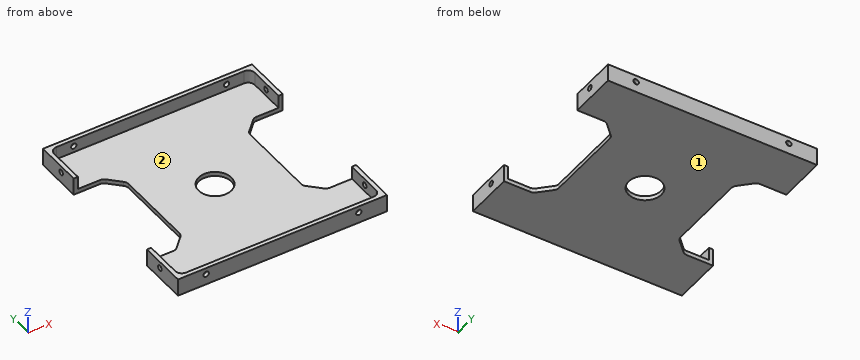
```python
from build123d import *

# Parameters (mm, degrees)
SKETCH1_W                      = 95.8
SKETCH1_H                      = 95.8
BOSS_EXTRUDE1_DEPTH            = 8
SKETCH2_W                      = 92
SKETCH2_H                      = 92
COMPONENT_PLATFORM_DEPTH       = 6
CABLE_SLOTS_DEPTH              = 6
SKETCH4_R                      = 7.5
CENTER_MASS_CUT_DEPTH          = 6
INNER_CORNER_FILLETS_R         = 3
M3X0_5_TAPPED_HOLE1_AT_2_COUNT = 2
M3X0_5_TAPPED_HOLE1_AT_2_PITCH = 70
M3X0_5_TAPPED_HOLE2_AT_2_COUNT = 2
M3X0_5_TAPPED_HOLE2_AT_2_PITCH = 70


with BuildPart() as part:
    # Sketch1 → Boss-Extrude1 (new body)
    with BuildSketch(Plane.XY):
        Rectangle(SKETCH1_W, SKETCH1_H)
    extrude(amount=BOSS_EXTRUDE1_DEPTH)

    # Sketch2 → Component Platform (cut)
    with BuildSketch(Plane.XY.offset(8)):
        Rectangle(SKETCH2_W, SKETCH2_H)
    extrude(amount=-COMPONENT_PLATFORM_DEPTH, mode=Mode.SUBTRACT)

    # Sketch3 → Cable Slots (cut, symmetric)
    with BuildSketch(Plane.XY.offset(2)):
        with BuildLine():
            Line((-33.778679656, -25.021320344), (-28.778679656, -20.021320344))
            ThreePointArc((-28.778679656, -20.021320344), (-28.128361402, -19.048050297), (-27.9, -17.9))
            Line((-27.9, -17.9), (-27.9, 18.1))
            ThreePointArc((-27.9, 18.1), (-28.128361402, 19.248050297), (-28.778679656, 20.221320344))
            Line((-28.778679656, 20.221320344), (-33.778679656, 25.221320344))
            ThreePointArc((-33.778679656, 25.221320344), (-34.751949703, 25.871638598), (-35.9, 26.1))
            Line((-35.9, 26.1), (-47.9, 26.1))
            Line((-47.9, 26.1), (-47.9, -25.9))
            Line((-47.9, -25.9), (-35.9, -25.9))
            ThreePointArc((-35.9, -25.9), (-34.751949703, -25.671638598), (-33.778679656, -25.021320344))
        make_face()
        with BuildLine():
            Line((47.9, -25.9), (47.9, 26.1))
            Line((47.9, 26.1), (35.9, 26.1))
            ThreePointArc((35.9, 26.1), (34.751949703, 25.871638598), (33.778679656, 25.221320344))
            Line((33.778679656, 25.221320344), (28.778679656, 20.221320344))
            ThreePointArc((28.778679656, 20.221320344), (28.128361402, 19.248050297), (27.9, 18.1))
            Line((27.9, 18.1), (27.9, -17.9))
            ThreePointArc((27.9, -17.9), (28.128361402, -19.048050297), (28.778679656, -20.021320344))
            Line((28.778679656, -20.021320344), (33.778679656, -25.021320344))
            ThreePointArc((33.778679656, -25.021320344), (34.751949703, -25.671638598), (35.9, -25.9))
            Line((35.9, -25.9), (47.9, -25.9))
        make_face()
    extrude(amount=CABLE_SLOTS_DEPTH, both=True, mode=Mode.SUBTRACT)

    # Sketch4 → Center Mass Cut (cut)
    with BuildSketch(Plane.XY.offset(2)):
        Circle(SKETCH4_R)
    extrude(amount=-CENTER_MASS_CUT_DEPTH, mode=Mode.SUBTRACT)

    # Inner Corner Fillets
    inner_corner_fillets_edges = [part.edges().sort_by_distance(p)[0] for p in [
        (-46, -46, 5),
        (-46, 46, 5),
        (46, 46, 5),
        (46, -46, 5),
    ]]
    fillet(inner_corner_fillets_edges, radius=INNER_CORNER_FILLETS_R)

    # Sketch10 → M3x0.5 Tapped Hole1 (revolve, cut)
    with BuildSketch(Plane(origin=(47.9, -35, 5), x_dir=(0, 0, -1), z_dir=(0, 1, 0))):
        Polygon((0, 0), (0, 10.751075774), (1.25, 10), (1.25, 0), align=None)
    m3x0_5_tapped_hole1 = revolve(axis=Axis((54.25, -35, 5), (-1, 0, 0)), mode=Mode.SUBTRACT)

    # M3x0.5 Tapped Hole1 at 2: M3x0.5 Tapped Hole1 ×2
    with Locations(*[(0, i * M3X0_5_TAPPED_HOLE1_AT_2_PITCH, 0) for i in range(1, M3X0_5_TAPPED_HOLE1_AT_2_COUNT)]):
        add(m3x0_5_tapped_hole1, mode=Mode.SUBTRACT)

    # Sketch13 → M3x0.5 Tapped Hole2 (revolve, cut)
    with BuildSketch(Plane(origin=(-35, -47.9, 5), x_dir=(0, 0, -1), z_dir=(1, 0, 0))):
        Polygon((0, 0), (0, 10.751075774), (1.25, 10), (1.25, 0), align=None)
    m3x0_5_tapped_hole2 = revolve(axis=Axis((-35, -54.25, 5), (0, 1, 0)), mode=Mode.SUBTRACT)

    # M3x0.5 Tapped Hole2 at 2: M3x0.5 Tapped Hole2 ×2
    with Locations(*[(i * M3X0_5_TAPPED_HOLE2_AT_2_PITCH, 0, 0) for i in range(1, M3X0_5_TAPPED_HOLE2_AT_2_COUNT)]):
        add(m3x0_5_tapped_hole2, mode=Mode.SUBTRACT)

    # Mirror1: M3x0.5 Tapped Hole1 across plane
    add(m3x0_5_tapped_hole1.mirror(Plane(origin=(-0.1, 0, 0), x_dir=(0, 0, 1), z_dir=(1, 0, 0))), mode=Mode.SUBTRACT)

    # Mirror1 copy 1 sketch → Mirror1 copy 1 (revolve, cut)
    with BuildSketch(Plane(origin=(-48.1, 35, 5), x_dir=(0, 0, -1), z_dir=(0, 1, 0))):
        Polygon((0, 0), (0, -10.751075774), (1.25, -10), (1.25, 0), align=None)
    revolve(axis=Axis((-54.45, 35, 5), (-1, 0, 0)), mode=Mode.SUBTRACT)

    # Mirror2: M3x0.5 Tapped Hole2 across plane
    add(m3x0_5_tapped_hole2.mirror(Plane(origin=(0, 0.1, 0), x_dir=(0, 0, 1), z_dir=(0, -1, 0))), mode=Mode.SUBTRACT)

    # Mirror2 copy 1 sketch → Mirror2 copy 1 (revolve, cut)
    with BuildSketch(Plane(origin=(35, 48.1, 5), x_dir=(0, 0, -1), z_dir=(1, 0, 0))):
        Polygon((0, 0), (0, -10.751075774), (1.25, -10), (1.25, 0), align=None)
    revolve(axis=Axis((35, 54.45, 5), (0, 1, 0)), mode=Mode.SUBTRACT)


solid = part.part
```
Source: CAD feature listing. Evaluate the final solid. Frame: model axes, mm. Face numbers are marked on the shaded views. Coordinates: 2 decimals unless noted, no trailing zeros. Write each loop counter-clockwise with the first axis right and the second up, starting at its lowest first coordinate (ties: lowest second). Pieces come first, ordered by that corner, then holes. Notation, with made-up numbers: (-25, 59.5) -> (32, 59.5) arc R33 ccw to (32, 94.5) -> close; hole circle Ø1 at (41, -14). An arc over 180 degrees is marked (long way). Return JSON: item names as keys, results as strings. Group by question number.
1) Section query A-A, the plane y = 0. Return loops of the section in (x, z).
2) Contact query for flat-ended pins moving along their axis: P1, Ø1.6, axis at y = -8, z = 1.5, coming from the +X side; P2, Ø1.5, axis at y = 35, z = 5, coming from the -X side; P3, Ø4, axis at x = -21, y = 20, coming from the -Z side. Output: stop coordinate, or through.
3) Section query D-D, the plane z = 5. State how many separate pieces and enclosed holes the cut face has, plus the area to 3 significant figures.
4) Section query B-B, the plane x = 0. Return loops of the section in (y, z), plus the area to 3 significant figures.
5) Section query C-C, the plane y = 35. Return loops of the section in (x, z).
6) Mould query, pull axis Y, two halves, no side actions, for the marked faces 1 and 2. Classes: +Y half, -Y half, draft (parallel to the pull), parting line (faces both ways), or undercut.
7) Ray query, line 1 along Y through (x, z) = (46.9, 5); line 2 along X through (y, z) = (-47.1, 5); line 3 along Y through (x, z) = (-13, 3.5). Return the intervals inside material, ascending.
From the geometry:
{
 "1": {"outline": "(-27.9, 0) -> (-7.5, 0) -> (-7.5, 2) -> (-27.9, 2) -> close; (7.5, 0) -> (27.9, 0) -> (27.9, 2) -> (7.5, 2) -> close"},
 "2": {"P1": "x = 27.9", "P2": "through", "P3": "z = 0"},
 "3": {"separate pieces": "10", "enclosed holes": "0", "area": "486 mm²"},
 "4": {"outline": "(-47.9, 0) -> (-7.5, 0) -> (-7.5, 2) -> (-46, 2) -> (-46, 8) -> (-47.9, 8) -> close; (7.5, 0) -> (47.9, 0) -> (47.9, 8) -> (46, 8) -> (46, 2) -> (7.5, 2) -> close", "area": "184 mm²"},
 "5": {"outline": "(-47.9, 0) -> (47.9, 0) -> (47.9, 3.75) -> (46, 3.75) -> (46, 2) -> (-46, 2) -> (-46, 3.75) -> (-47.9, 3.75) -> close; (-47.9, 6.25) -> (-46, 6.25) -> (-46, 8) -> (-47.9, 8) -> close; (46, 6.25) -> (47.9, 6.25) -> (47.9, 8) -> (46, 8) -> close"},
 "6": {"face 1": "draft", "face 2": "undercut"},
 "7": {"line 1": "-47.9 to -36.25, -33.75 to -25.9, 26.1 to 33.75, 36.25 to 47.9", "line 2": "-47.9 to -36.25, -33.75 to 33.75, 36.25 to 47.9", "line 3": "-47.9 to -46, 46 to 47.9"}
}
